from build123d import *

# Parameters (mm, degrees)
F0_R     = 19.685
F1_DEPTH = 38.1
F2_R     = 25.4
F3_DEPTH = 1.5875
F6_D     = 7.9375


with BuildPart() as f1:
    # F0 (on Right) → F1 (new body, symmetric)
    with BuildSketch(Plane.YZ):
        Circle(F0_R)
    extrude(amount=F1_DEPTH, both=True)

    # F2 (on Right) → F3 (join, symmetric)
    with BuildSketch(Plane.YZ):
        Circle(F2_R)
    extrude(amount=F3_DEPTH, both=True)

    # F6 (through all)
    with Locations(Plane.XY.offset(25.4)):
        with Locations((-20.6375, 0), (20.6375, 0)):
            Hole(F6_D / 2)


solid = f1.part
Geometry check sheet. Reference: the model listing, model coordinates, mm. A direction names the side the tool comes from. Coordinates: 2 decimals unless noted, no trailing zeros. Order: outer loops, then holes, each group sorted by start corner. A loop starts at its lowest first (then second) coordinate and runs counter-clockwise, first axis right, second up. Notation, with made-up numbers: (45.5, -27.75) - (60.5, -27.75) arc R6 cw to (60.5, -19.75) - close; hole circle Ø6 at (37, 54). An arc over 180 degrees is marked (long way). One line per item, written item: value.
(1) Release check for a two-part mould opening along Y. For faces 1 (the face through (0.022, -5.506, -24.796)), 2 (the face through (-24.304, -1.52, -0.276)), 3 (the face through (38.1, 0, 0)) record: +Y half, -Y half, draft (parallel to the pull), parting line (faces both ways), or undercut.
Data:
face 1: parting line
face 2: undercut
face 3: draft
(2) Depth check by flat-ended pin: pin 1 Ø8 at (x, z) = (-9.5, 2.5) entering from +Y (3 decimals); pin 2 Ø9 at (x, y) = (20.64, 0) entering from +Z (3 decimals); pin 3 Ø5 at (x, y) = (-27, 18) entering from +Z. Enter the tip coordinate at first touch or a pass-through.
Data:
pin 1: stops at y = 19.685
pin 2: stops at z = 19.685
pin 3: stops at z = 12.13
(3) Access from +Z, -Z, +X, -X, +Y, -Y to the whole of each face (thin tool, end or side, straight path). Record for faces 4 (the face through (24.6, 0.2, -0.3)), 5 (the face through (1.588, 13, -15)), 6 (the face through (-19.588, -4.267, -19.217)).
Data:
face 4: +Z, -Z
face 5: +X
face 6: -X
(4) Sectioned sample at D-D (y = -12). Enter the section's corners in (x, z), and give its area (3 significant figures).
Data:
outline: (-38.1, -15.6) - (-1.59, -15.6) - (-1.59, -22.39) - (1.59, -22.39) - (1.59, -15.6) - (38.1, -15.6) - (38.1, 15.6) - (1.59, 15.6) - (1.59, 22.39) - (-1.59, 22.39) - (-1.59, 15.6) - (-38.1, 15.6) - close
area: 2,420 mm^2
(5) Sectioned sample at B-B (z = 0). Enter the section's corners in (x, y) (1 decimal), and give its area (3 significant figures).
Data:
outline: (-38.1, -19.7) - (-1.6, -19.7) - (-1.6, -25.4) - (1.6, -25.4) - (1.6, -19.7) - (38.1, -19.7) - (38.1, 19.7) - (1.6, 19.7) - (1.6, 25.4) - (-1.6, 25.4) - (-1.6, 19.7) - (-38.1, 19.7) - close; hole circle Ø7.9 at (-20.6, 0); hole circle Ø7.9 at (20.6, 0)
area: 2,940 mm^2
(6) Sectioned sample at A-A (y = 0). Enter the section's corners in (x, z) (1 decimal), and give its area (3 significant figures).
Data:
outline: (-38.1, -19.7) - (-24.6, -19.7) - (-24.6, 19.7) - (-38.1, 19.7) - close; (-16.7, -19.7) - (-1.6, -19.7) - (-1.6, -25.4) - (1.6, -25.4) - (1.6, -19.7) - (16.7, -19.7) - (16.7, 19.7) - (1.6, 19.7) - (1.6, 25.4) - (-1.6, 25.4) - (-1.6, 19.7) - (-16.7, 19.7) - close; (24.6, -19.7) - (38.1, -19.7) - (38.1, 19.7) - (24.6, 19.7) - close
area: 2,410 mm^2
(7) Sectioned sample at C-C (z = -17.5). Enter the section's corners in (x, y), and give its area (3 significant figures).
Data:
outline: (-38.1, -9.01) - (-1.59, -9.01) - (-1.59, -18.41) - (1.59, -18.41) - (1.59, -9.01) - (38.1, -9.01) - (38.1, 9.01) - (1.59, 9.01) - (1.59, 18.41) - (-1.59, 18.41) - (-1.59, 9.01) - (-38.1, 9.01) - close; hole circle Ø7.94 at (-20.64, 0); hole circle Ø7.94 at (20.64, 0)
area: 1,330 mm^2
(8) Thickness scan on probe 1 along X at (y, z) = (0, -6.5); probe 2 along X at (y, z) = (-1, 7.5); probe 3 along X at (y, z) = (-16, -14). Record the ranges inside material, lowest first. Write a range as from..to.
Data:
probe 1: x = -38.1..-24.61, -16.67..16.67, 24.61..38.1
probe 2: x = -38.1..-24.48, -16.8..16.8, 24.48..38.1
probe 3: x = -1.59..1.59
